```python
from build123d import *

# Parameters (mm, degrees)
SKETCH_R        = 15
PAD_DEPTH       = 5.5
SKETCH001_R     = 4.5
SKETCH001_R_2   = 1.6
POCKET_DEPTH    = 5.501
SKETCH002_R     = 11.25
POCKET001_DEPTH = 2.5
SKETCH003_R     = 3
POCKET002_DEPTH = 2


with BuildPart() as part:
    # Sketch → Pad (new body)
    with BuildSketch(Plane.XY):
        Circle(SKETCH_R)
    extrude(amount=PAD_DEPTH)

    # Sketch001 (on Face3 of Pad) → Pocket (cut, through all)
    with BuildSketch(Plane.XY.offset(5.5)):
        Circle(SKETCH001_R)
        with Locations((0, 8.5)):
            Circle(SKETCH001_R_2)
        with Locations((0, -8.5)):
            Circle(SKETCH001_R_2)
    extrude(amount=-POCKET_DEPTH, mode=Mode.SUBTRACT)

    # Sketch002 (on Face3 of Pocket) → Pocket001 (cut)
    with BuildSketch(Plane.XY.offset(5.5)):
        Circle(SKETCH002_R)
    extrude(amount=-POCKET001_DEPTH, mode=Mode.SUBTRACT)

    # Sketch003 (on Face2 of Pocket001) → Pocket002 (cut)
    with BuildSketch(Plane(origin=(0, 0, 0), x_dir=(1, 0, 0), z_dir=(0, 0, -1))):
        with Locations((0, 8.5)):
            Circle(SKETCH003_R)
        with Locations((0, -8.5)):
            Circle(SKETCH003_R)
    extrude(amount=-POCKET002_DEPTH, mode=Mode.SUBTRACT)


solid = part.part
```
Here's how the part is built. I have some questions about the finished solid (model axes, mm). A direction names the side the tool comes from. Give positions to 0.01 mm unless a question says otherwise; leave off trailing zeros. Order: outer loops, then holes, each group sorted by start corner. A loop starts at its lowest first (then second) coordinate and runs counter-clockwise, first axis right, second up. Notation, with made-up numbers: (36.5, 9) - (58.5, 9) arc R11 cw to (58.5, 13) - close; hole circle Ø8 at (-9.75, -24). An arc over 180 degrees is marked (long way). Answer as a JSON object with one key per item and string values. Group by question number.
Item 1: If we mould it in two halves opening along X, with no side actions, what happens to faces 4 (the cylindrical face through (-14.985, 0.66, 2.712)), 5 (the cylindrical face through (-0.35, -10.06, 2.51)), 6 (the flat face through (3, 4, 0))? For each: pulls with the +X half, pulls with the -X half, needs draft (parallel to the pull), parting line crosses it, or undercut.
Item 2: For P1, Ø1.5, axis at x = -1, z = 2.5, coming from the +Y side; P2, Ø3, axis at y = -7, z = 2, coming from the +X side; P3, Ø3.5, axis at x = 0, y = 8.5, coming from the +Z side; P4, Ø3, axis at x = 0, y = -8.5, coming from the -Z side, each with a flat end and sliding along its axis, tell me the tip position at first contact or that it passes through.
Item 3: If we section it at A-A on y = -1: Please give me the cut outline in (x, z), and give its area (3 significant figures).
Item 4: Please list where these lines run through material, in increasing order: probe 1 along Y at (x, z) = (0, 1.35); probe 2 along Y at (x, z) = (0, 2.2); probe 3 along X at (y, z) = (0.25, 4.8).
Item 5: If we section it at D-D on y = 7.5: Please give me the cut outline in (x, z).
Item 6: If we section it at B-B on x = 0: Please give me the cut outline in (y, z), and give its area (4 significant figures).
Item 7: If we section it at C-C on z = 4.8: Please give me the cut outline in (x, y).
Item 8: Which directions (+Z, -Z, +X, -X, +Y, -Y) give clear straight access to the entire face, cutting with the end or side of a thin tool? Please do faces 1 (the cylindrical face through (-0.35, 6.94, 2.51)), 2 (the cylindrical face through (-0.391, 5.526, 0.986)), 3 (the flat face through (5, 0, 3)).
Result set:
{
 "1": {"face 4": "parting line crosses it", "face 5": "undercut", "face 6": "needs draft"},
 "2": {"P1": "y = 15", "P2": "x = 13.96", "P3": "z = 3", "P4": "through"},
 "3": {"outline": "(-14.97, 0) - (-4.39, 0) - (-4.39, 3) - (-11.21, 3) - (-11.21, 5.5) - (-14.97, 5.5) - close; (4.39, 0) - (14.97, 0) - (14.97, 5.5) - (11.21, 5.5) - (11.21, 3) - (4.39, 3) - close", "area": "82.3 mm²"},
 "4": {"probe 1": "-15 to -11.5, -5.5 to -4.5, 4.5 to 5.5, 11.5 to 15", "probe 2": "-15 to -10.1, -6.9 to -4.5, 4.5 to 6.9, 10.1 to 15", "probe 3": "-15 to -11.25, 11.25 to 15"},
 "5": {"outline": "(-12.99, 0) - (-2.83, 0) - (-2.83, 2) - (-1.25, 2) - (-1.25, 3) - (-8.39, 3) - (-8.39, 5.5) - (-12.99, 5.5) - close; (1.25, 2) - (2.83, 2) - (2.83, 0) - (12.99, 0) - (12.99, 5.5) - (8.39, 5.5) - (8.39, 3) - (1.25, 3) - close"},
 "6": {"outline": "(-15, 0) - (-11.5, 0) - (-11.5, 2) - (-10.1, 2) - (-10.1, 3) - (-11.25, 3) - (-11.25, 5.5) - (-15, 5.5) - close; (-6.9, 2) - (-5.5, 2) - (-5.5, 0) - (-4.5, 0) - (-4.5, 3) - (-6.9, 3) - close; (4.5, 0) - (5.5, 0) - (5.5, 2) - (6.9, 2) - (6.9, 3) - (4.5, 3) - close; (10.1, 2) - (11.5, 2) - (11.5, 0) - (15, 0) - (15, 5.5) - (11.25, 5.5) - (11.25, 3) - (10.1, 3) - close", "area": "51.35 mm²"},
 "7": {"outline": "circle Ø30 at (0, 0); hole circle Ø22.5 at (0, 0)"},
 "8": {"face 1": "+Z, -Z", "face 2": "-Z", "face 3": "+Z"}
}
